For this review, take the finished solid that the model builds, in its own axes (mm). Face numbers are marked on the shaded views. A direction names the side the tool comes from. Coordinates: 2 decimals unless noted, no trailing zeros. Write each loop counter-clockwise with the first axis right and the second up, starting at its lowest first coordinate (ties: lowest second). Pieces come first, ordered by that corner, then holes. Notation, with made-up numbers: M -21.75,-2 L -13.75,-2 A33 ccw -13.75,35 Z; hole C 8,11.5 d3. An arc over 180 degrees is marked long. One line per question, with ' | ' between items.
from build123d import *

# Parameters (mm, degrees)
F0_W          = 203.2
F0_H          = 127
F1_DEPTH      = 127
F3_DEPTH      = 76.2
F3_DEPTH_BACK = 76.2
F4_DEPTH      = 25.4
F5_SIZE2      = 101.6
F5_SIZE       = 76.2
F6_R          = 5.08
F7_R          = 15.24
F8_DEPTH      = 51.054
F9_R          = 15.24
F10_DEPTH     = 128.27


with BuildPart() as f1:
    # F0 (on Front) → F1 (new body)
    with BuildSketch(Plane.XZ):
        Rectangle(F0_W, F0_H)
    extrude(amount=F1_DEPTH)

    # F2 (on Front) → F3 (cut, two sides)
    with BuildSketch(Plane.XZ) as f3_sk:
        Polygon((25.2138410211, 63.1450035885), (-101.7861589789, 63.1450035885), (-101.7861589789, -63.8549964115), (-25.5861589789, -63.8549964115), (-25.5861589789, 12.3450035885), (25.2138410211, 12.3450035885), align=None)
    extrude(amount=-F3_DEPTH, mode=Mode.SUBTRACT)
    extrude(f3_sk.sketch, amount=F3_DEPTH_BACK, mode=Mode.SUBTRACT)

    # F4 (cut): a face of the model
    f4_faces = [f1.faces().sort_by_distance(p)[0] for p in [
        (-38.1930794895, -38.1, 63.1450035885),
    ]]
    extrude(f4_faces, amount=-F4_DEPTH, mode=Mode.SUBTRACT)

    # F5
    f5_edges = [f1.edges().sort_by_distance(p)[0] for p in [
        (-101.6, -101.6, 63.5),
    ]]
    f5_side = f1.faces().sort_by_distance((-101.6, -101.6, 0))[0]
    chamfer(f5_edges, length=F5_SIZE, length2=F5_SIZE2, reference=f5_side)

    # F6
    f6_edges = [f1.edges().sort_by_distance(p)[0] for p in [
        (25.213841, 0, 37.922502),
        (63.406921, 0, 63.5),
        (-0.186159, 0, 12.345004),
        (-25.586159, -38.1, 12.345004),
        (-101.6, -101.6, -12.7),
        (0, -101.6, 63.5),
        (101.6, 0, 0),
        (38.006921, 0, -63.5),
        (-25.586159, -38.1, -63.5),
        (-63.593079, -76.2, -63.5),
        (-101.6, -101.6, -63.5),
        (50.8, -127, 63.5),
        (-50.8, -127, 25.4),
        (101.6, -127, 0),
        (-101.6, -127, -38.1),
        (0, -127, -63.5),
        (-50.8, -76.2, 25.4),
        (101.6, -63.5, 63.5),
        (101.6, -63.5, -63.5),
        (12.606921, -76.2, 63.5),
        (25.213841, -38.1, 63.5),
    ]]
    fillet(f6_edges, radius=F6_R)

    # F7 (on face) → F8 (cut)
    with BuildSketch(Plane(origin=(0, -76.2, 0), x_dir=(-1, 0, 0), z_dir=(0, 1, 0))):
        with Locations((64.0217885375, -31.3331931829)):
            Circle(F7_R)
    extrude(amount=-F8_DEPTH, mode=Mode.SUBTRACT)

    # F9 (on face) → F10 (cut)
    with BuildSketch(Plane.XY.offset(63.5)):
        with Locations((69.9954107404, -40.2551107109)):
            Circle(F9_R)
    extrude(amount=-F10_DEPTH, mode=Mode.SUBTRACT)


solid = f1.part
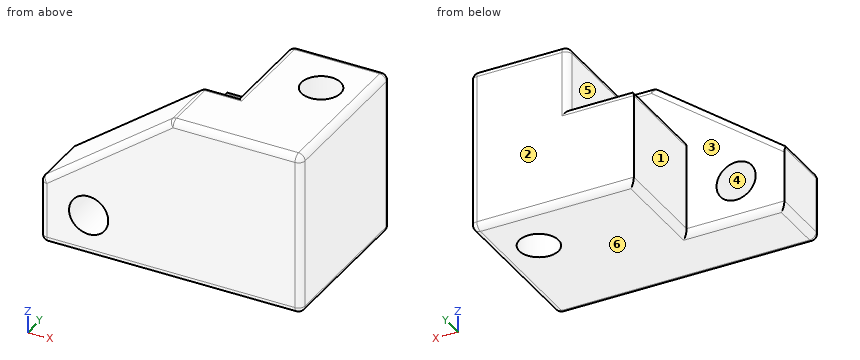
1) Machinability: for the marked faces 1, 2 and 3, which of the approach directions +Z, -Z, +X, -X, +Y, -Y give a long, thin tool a straight path to every point of the face, cutting with its end or side? Answer none if there is none.
Responses:
face 1: +Z, -Z, -X, +Y | face 2: +Z, -Z, +X, -X, +Y | face 3: +Z, -X, +Y
2) To check wall thickness, follow line 1 along X through (y, z) = (-23.5, -25.5); line 2 along Y through (x, z) = (-79.5, -6); line 3 along X through (y, z) = (-51.5, -36). State the ranges of each line that lie inside material, in increasing order. Write a range as [from, to].
Responses:
line 1: [-25.59, 101.6] | line 2: [-127, -76.2] | line 3: [-25.59, 59.71], [80.28, 101.6]
3) The part is to be moulded in two halves that separate along X. For the marked faces 4, 5 and 6, say which applies: +X half, -X half, draft (parallel to the pull), parting line (faces both ways), or undercut.
Responses:
face 4: undercut | face 5: -X half | face 6: draft
4) We need section C-C on y = -104.5. State the section outline as (x, z) points.
Responses:
outline: M -101.6,-58.42 A5.08 ccw -96.52,-63.5 L 96.52,-63.5 A5.08 ccw 101.6,-58.42 L 101.6,58.42 A5.08 ccw 96.52,63.5 L 1.69,63.5 A5.08 ccw -1.35,62.48 L -99.57,-11.18 A5.08 ccw -101.6,-15.24 Z; hole C -64.02,-31.33 d30.48
5) Insertion check: pin 1 Ø23 at (x, y) = (7.5, -42) entering from +Z (3 decimals); pin 2 Ø24.5 at (x, y) = (70, -40.26) entering from +Z; pin 3 Ø14 at (y, z) = (-37, 44) entering from -X. Each pin has a flat end and moves straight along its axis. Give the tip position at first contact, or say it passes through.
Responses:
pin 1: z = 12.345 | pin 2: through | pin 3: x = 25.21
6) We need section A-A on y = -20.5. State the section outline as (x, z) points (3 decimals), then the cut area to 3 significant figures.
Responses:
outline: M -25.586,-58.42 A5.08 ccw -20.506,-63.5 L 96.52,-63.5 A5.08 ccw 101.6,-58.42 L 101.6,58.42 A5.08 ccw 96.52,63.5 L 30.294,63.5 A5.08 ccw 25.214,58.42 L 25.214,12.345 L -20.506,12.345 A5.08 ccw -25.586,7.265 Z | area: 13,500 mm^2
7) We need section B-B on x = 11. State the section outline as (y, z) points (3 decimals).
Responses:
outline: M -127,-58.42 A5.08 ccw -121.92,-63.5 L -5.08,-63.5 A5.08 ccw 0,-58.42 L 0,7.265 A5.08 ccw -5.08,12.345 L -76.2,12.345 L -76.2,58.42 A5.08 ccw -81.28,63.5 L -121.92,63.5 A5.08 ccw -127,58.42 Z
